Build history of the part. All positions in model axes, mm. A direction names the side the tool comes from. Coordinates: 2 decimals unless noted, no trailing zeros. Loops run counter-clockwise (first coordinate to the right, second up) from the corner with the lowest first, then second, coordinate; pieces in that order, holes last. Notation, with made-up numbers: (-7.5, -12) - (39.5, -12) arc R21 cw to (39.5, 24) - close; hole circle Ø6 at (78.25, 50). An arc over 180 degrees is marked (long way). One line per item, written item: value.
```python
from build123d import *

# Parameters (mm, degrees)
SKETCH_1_W          = 70
SKETCH_1_H          = 40
EXTRUDE_1_DEPTH     = 18
SKETCH_3_W          = 70
SKETCH_3_H          = 6.5
EXTRUDE_2_DEPTH     = 59
SKETCH_4_W          = 15
SKETCH_4_H          = 15
EXTRUDE_3_DEPTH     = 6.5
SKETCH_5_W          = 10
SKETCH_5_H          = 5
EXTRUDE_4_DEPTH     = 80
SKETCH_7_R          = 4
CUT_EXTRUDE_1_DEPTH = 18


with BuildPart() as part:
    # 草图1 → 凸台-拉伸1 (new body)
    with BuildSketch(Plane(origin=(0, 0, 0), x_dir=(1, 0, 0), z_dir=(0, 1, 0))):
        with Locations((35, -20)):
            Rectangle(SKETCH_1_W, SKETCH_1_H)
    extrude(amount=EXTRUDE_1_DEPTH)

    # 草图3 → 凸台-拉伸2 (add)
    with BuildSketch(Plane(origin=(0, 18, 0), x_dir=(1, 0, 0), z_dir=(0, 1, 0))):
        with Locations((35, -43.25)):
            Rectangle(SKETCH_3_W, SKETCH_3_H)
    extrude(amount=-EXTRUDE_2_DEPTH)

    # 草图4 → 凸台-拉伸3 (add)
    with BuildSketch(Plane.XY.offset(46.5)):
        with Locations((-7.5, -33.5)):
            Rectangle(SKETCH_4_W, SKETCH_4_H)
    extrude_3 = extrude(amount=-EXTRUDE_3_DEPTH)

    # 镜向1: 凸台-拉伸3 across plane
    add(extrude_3.mirror(Plane(origin=(35, 0, 0), x_dir=(0, 0, 1), z_dir=(1, 0, 0))))

    # 草图5 → 凸台-拉伸4 (add)
    with BuildSketch(Plane.XY.offset(46.5)):
        with Locations((-10, -38.5)):
            Rectangle(SKETCH_5_W, SKETCH_5_H)
    extrude_4 = extrude(amount=EXTRUDE_4_DEPTH)

    # 镜向2: 凸台-拉伸4 across plane
    add(extrude_4.mirror(Plane(origin=(35, 0, 0), x_dir=(0, 0, 1), z_dir=(1, 0, 0))))

    # 草图7 → 切除-拉伸1 (cut)
    with BuildSketch(Plane(origin=(0, 18, 0), x_dir=(1, 0, 0), z_dir=(0, 1, 0))):
        with Locations(Location((35, -18.523, 0), (0, 0, 270))):
            Circle(SKETCH_7_R)
        with Locations(Location((60, -18.523, 0), (0, 0, 270))):
            Circle(SKETCH_7_R)
        with Locations(Location((10, -18.523, 0), (0, 0, 270))):
            Circle(SKETCH_7_R)
    extrude(amount=-CUT_EXTRUDE_1_DEPTH, mode=Mode.SUBTRACT)


solid = part.part
```
Item 1: Drop flat-ended pins along their axis: P1, Ø3, axis at x = 47.5, y = -32, coming from the +Z side; P2, Ø7, axis at x = -9, z = 43.5, coming from the +Y side; P3, Ø11, axis at x = 79.5, z = 67.5, coming from the +Y side. Give the stop position or say it passes through.
Check result:
P1: stops at z = 46.5
P2: stops at y = -26
P3: stops at y = -36
Item 2: Cut at C-C, the plane y = 2. Write the cut outline in (x, z).
Check result:
outline: (0, 0) - (70, 0) - (70, 46.5) - (0, 46.5) - close; hole circle Ø8 at (10, 18.52); hole circle Ø8 at (35, 18.52); hole circle Ø8 at (60, 18.52)
Item 3: Pull direction Z, two halves, no side cores. Call faces 1 (the face through (38.966, 9.126, 18.002)), 2 (the face through (36, -20, 40)), 3 (the face through (80, -38, 126.5)), 4 (the face through (-8, -26, 43)): released by +Z, released by -Z, zero draft, split by the parting line, or undercut.
Check result:
face 1: undercut
face 2: released by -Z
face 3: released by +Z
face 4: zero draft
Item 4: Cut at B-B, the plane x = 10. Write the cut outline in (y, z), then the cut area to 4 significant figures.
Check result:
outline: (-41, 40) - (0, 40) - (0, 22.52) - (18, 22.52) - (18, 46.5) - (-41, 46.5) - close; (0, 0) - (18, 0) - (18, 14.52) - (0, 14.52) - close
area: 959.5 mm^2
Item 5: Probe probe 1 along X at (y, z) = (-37.5, 104); probe 2 along Z at (x, y) = (16, 16.5); probe 3 along Z at (x, y) = (20, -31). List the from-to ranges inside material, lowest first. Write a range as from..to.
Check result:
probe 1: x = -15..-5, 75..85
probe 2: z = 0..46.5
probe 3: z = 40..46.5
Item 6: Cut at D-D, the plane z = 44.5. Write the cut outline in (x, y), then the cut area to 3 significant figures.
Check result:
outline: (-15, -41) - (85, -41) - (85, -26) - (70, -26) - (70, 18) - (0, 18) - (0, -26) - (-15, -26) - close
area: 4,580 mm^2
Item 7: Cut at A-A, the plane z = 102. Write the cut outline in (x, y), then the cut area to 3 significant figures.
Check result:
outline: (-15, -41) - (-5, -41) - (-5, -36) - (-15, -36) - close; (75, -41) - (85, -41) - (85, -36) - (75, -36) - close
area: 100 mm^2
Item 8: Tool access for faces 5 (the face through (0, 6, 24)), 6 (the face through (-5, -39, 86)), 7 (the face through (35, 0, 24)), 8 (the face through (-10, -36, 86)): list every direction of +Z, -Z, +X, -X, +Y, -Y with a clear straight run to the whole face (end or side of a thin tool).
Check result:
face 5: +Z, -Z, -X, +Y
face 6: +Z, +Y, -Y
face 7: -Z, +X, -X, -Y
face 8: +Z, +X, -X, +Y
